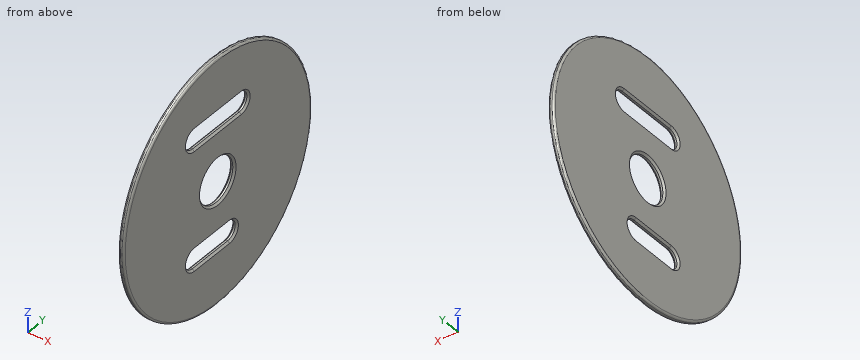
Autodesk Inventor part; units mm, degrees
ref_plane "YZ Plane" through (0, 0, 0) normal (1, 0, 0) x (0, 1, 0)
ref_plane "XZ Plane" through (0, 0, 0) normal (0, 1, 0) x (-1, 0, 0)
ref_plane "XY Plane" through (0, 0, 0) normal (0, 0, 1) x (1, 0, 0)
sketch "Sketch1" plane through (0, 0, 0) normal (1, 0, 0) x (0, 1, 0)
  circle A0 centre (0, 0) radius 3.6
  line L0 (-5, -9.75) -> (5, -9.75)
  line L1 (5, -9.75) -> (5, 9.75)
  line L2 (5, 9.75) -> (-5, 9.75)
  line L3 (-5, 9.75) -> (-5, -9.75)
  line L4 (-5, -9.75) -> (5, 9.75) construction
  line L5 (5, -9.75) -> (-5, 9.75) construction
  line L6 (5, 9.75) -> (-5, 9.75) construction
  line L7 (5, 11.35) -> (-5, 11.35)
  line L8 (-5, 8.15) -> (5, 8.15)
  arc A1 (5, 8.15) -> (5, 11.35) centre (5, 9.75) ccw
  arc A2 (-5, 11.35) -> (-5, 8.15) centre (-5, 9.75) ccw
  line L9 (-5, -9.75) -> (2.5, -9.75) construction
  line L10 (-5, -11.35) -> (2.5, -11.35)
  line L11 (2.5, -8.15) -> (-5, -8.15)
  arc A3 (-5, -8.15) -> (-5, -11.35) centre (-5, -9.75) ccw
  arc A4 (2.5, -11.35) -> (2.5, -8.15) centre (2.5, -9.75) ccw
  circle A5 centre (0, 0) radius 20
  point P0 (0, 9.75)
  point P1 (-1.25, -9.75)
  dimension "d0" = 7.2
  dimension "d1" = 19.5
  dimension "d2" = 10
  dimension "d3" = 1.6
  dimension "d4" = 7.5
  dimension "d5" = 40
  dimension "d12" = 1.6
extrude "Extrusion1" add sketch "Sketch1" along normal blind 0.9 contours A4 L11 L3 L8 L1 L0 | A5
fillet "Fillet1" radius 0.3 2 edges at (0.9, -20, 0) (0, -20, 0)
chamfer "Chamfer1" distance 0.3 angle 45 18 edges at (0.9, 0, 8.15) (0.9, -6.6, 9.75) (0.9, 0, 11.35) (0.9, 6.6, 9.75) (0.9, -3.6, 0) (0, -3.6, 0) (0, -1.25, -11.35) (0, -6.6, -9.75) (0, -1.25, -8.15) (0, 4.1, -9.75) (0.9, -1.25, -11.35) (0.9, -6.6, -9.75) (0.9, -1.25, -8.15) (0.9, 4.1, -9.75) (0, 0, 8.15) (0, -6.6, 9.75) (0, 0, 11.35) (0, 6.6, 9.75)
properties part number "CameraModuleSymbolDisc"
Geometry: final body of the model. Coordinates: model frame, mm. Coordinates: 2 decimals unless noted, no trailing zeros. Order: outer loops, then holes, each group sorted by start corner. A loop starts at its lowest first (then second) coordinate and runs counter-clockwise, first axis right, second up. Notation, with made-up numbers: (-36, 84) -> (-1, 84) arc R34 cw to (-1, 122) -> close; hole circle Ø10 at (50, -2.5). An arc over 180 degrees is marked (long way). Write each question's results on one line, items separated by ' | '. Start each with the question number.
1) Cut plane A-A, the plane y = 0. State how many separate pieces and enclosed holes the cut face has, and give its area (3 significant figures).
2) Material intervals for line 1 along Z through (x, y) = (0.45, 0); line 2 along Y through (x, z) = (0.25, 8.5); line 3 along Z through (x, y) = (0.6, -1), sorted ascending.
3) Cut plane C-C, the plane z = 0. Output: boundary loops of the cut face in (x, y).
4) Cut plane B-B, the plane x = 0.45. Output: boundary loops of the cut face in (y, z), and give its area (3 significant figures).
Checks:
1) separate pieces: 4 | enclosed holes: 0 | area: 23.1 mm^2
2) line 1: -20 to -11.35, -8.15 to -3.6, 3.6 to 8.15, 11.35 to 20 | line 2: -18.1 to -6.08, 6.08 to 18.1 | line 3: -19.97 to -11.35, -8.15 to -3.46, 3.46 to 8.15, 11.35 to 19.97
3) outline: (0, -19.7) arc R0.3 ccw to (0.3, -20) -> (0.6, -20) arc R0.3 ccw to (0.9, -19.7) -> (0.9, -3.9) -> (0.6, -3.6) -> (0.3, -3.6) -> (0, -3.9) -> close; (0, 3.9) -> (0.3, 3.6) -> (0.6, 3.6) -> (0.9, 3.9) -> (0.9, 19.7) arc R0.3 ccw to (0.6, 20) -> (0.3, 20) arc R0.3 ccw to (0, 19.7) -> close
4) outline: circle Ø40 at (0, 0); hole (-5, -11.35) -> (2.5, -11.35) arc R1.6 ccw to (2.5, -8.15) -> (-5, -8.15) arc R1.6 ccw to start; hole (-5, 8.15) -> (5, 8.15) arc R1.6 ccw to (5, 11.35) -> (-5, 11.35) arc R1.6 ccw to start; hole circle Ø7.2 at (0, 0) | area: 1,140 mm^2
